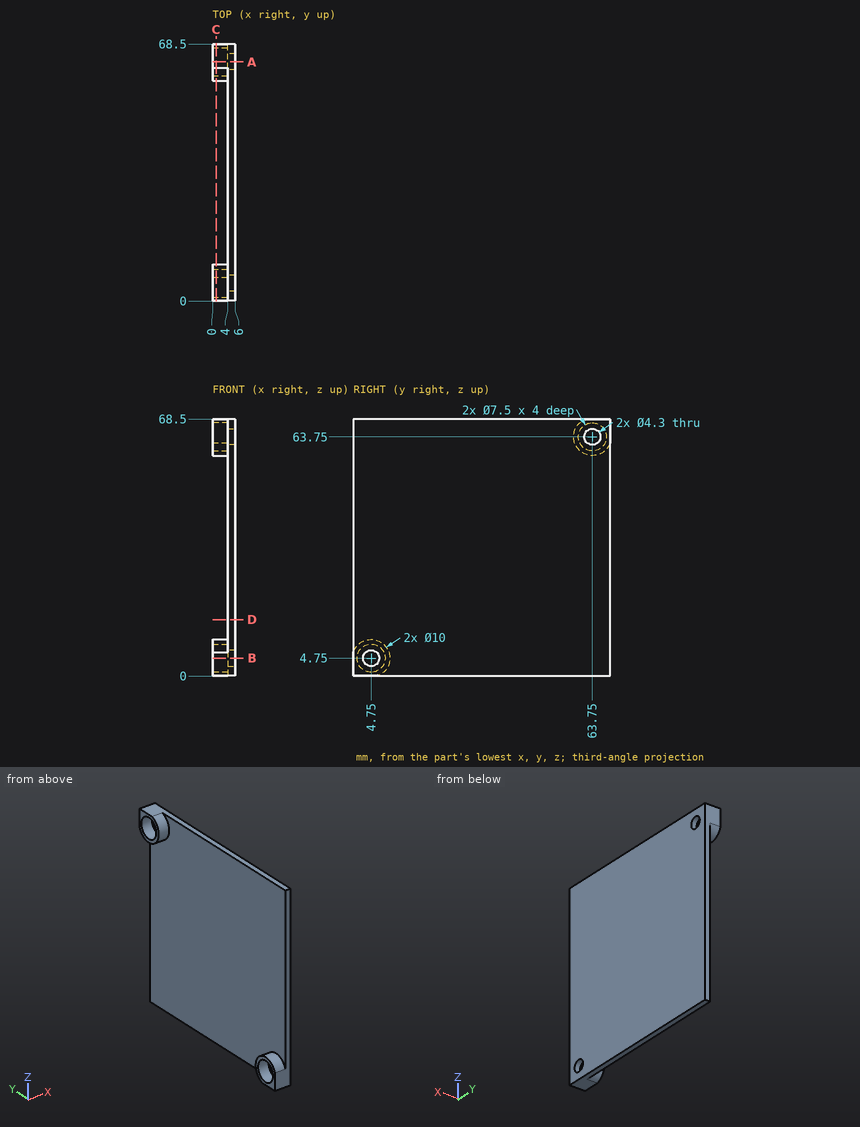
Study the drawing (mm; zero at the part's minimum x, y, z) and answer. Coordinates: 2 decimals unless noted, no trailing zeros. Write each loop counter-clockwise with the first axis right and the second up, starting at its lowest first coordinate (ties: lowest second). Pieces come first, ordered by that corner, then holes.
Q1. Section A-A, the plane y = 63.75 is taken. Write down the section's boundary in (x, z), then the cut area to 3 significant figures.
Returned:
outline: (0, 58.75) - (4, 58.75) - (4, 0) - (6, 0) - (6, 61.6) - (4, 61.6) - (4, 60) - (0, 60) - close; (0, 67.5) - (4, 67.5) - (4, 65.9) - (6, 65.9) - (6, 68.5) - (0, 68.5) - close
area: 137 mm2
Q2. Section B-B, the plane z = 4.75 is taken. Write down the section's boundary in (x, y), then the cut area to 3 significant figures.
Returned:
outline: (0, 0) - (6, 0) - (6, 2.6) - (4, 2.6) - (4, 1) - (0, 1) - close; (0, 8.5) - (4, 8.5) - (4, 6.9) - (6, 6.9) - (6, 68.5) - (4, 68.5) - (4, 9.75) - (0, 9.75) - close
area: 137 mm2
Q3. Section C-C, the plane x = 0.9 is taken. Write down the section's boundary in (y, z).
Returned:
outline: (0, 0) - (6.31, 0) arc R5 ccw (long way) to (0, 6.31) - close; (62.19, 68.5) arc R5 ccw (long way) to (68.5, 62.19) - (68.5, 68.5) - close; hole circle Ø7.5 at (4.75, 4.75); hole circle Ø7.5 at (63.75, 63.75)
Q4. Find the intervals of material crossed by line 1 along Y through (x, z) = (5.35, 4.75); line 2 along Z through (x, y) = (4.5, 4.5); line 3 along X through (y, z) = (7, 32), in increasing order.
Returned:
line 1: y = 0 to 2.6, 6.9 to 68.5
line 2: z = 0 to 2.61, 6.89 to 68.5
line 3: x = 4 to 6
Q5. Section D-D, the plane z = 15 is taken. Write down the section's boundary in (x, y).
Returned:
outline: (4, 0) - (6, 0) - (6, 68.5) - (4, 68.5) - close
Q6. Given P1, Ø3, axis at x = 1.5, z = 54, coming from the -Y side, flat-ended and moving along its own axis, determine where the tip first touches the part or whether it passes through.
Returned:
P1: passes through
